Verification items for this drawing (mm, ordinates from the low corner). Give positions to 0.01 mm unless a question says otherwise; leave off trailing zeros. Loops run counter-clockwise (first coordinate to the right, second up) from the corner with the lowest first, then second, coordinate; pieces in that order, holes last. Notation, with made-up numbers: M 1,44 L 29,44 A15 ccw 29,68 Z; hole C 48.5,14.25 d7. An arc over 180 degrees is marked long. Use one line per item in the form item = value.
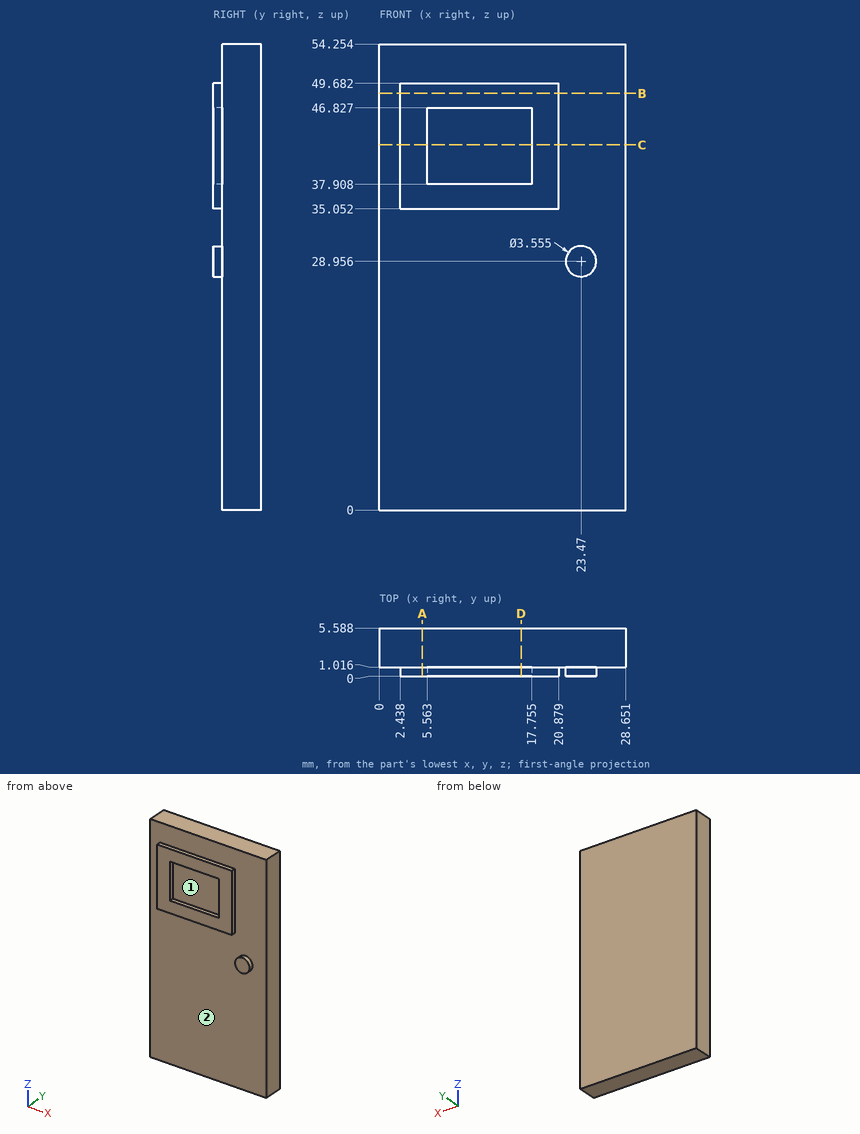
1) Section check C-C (z = 42.5). Record the cut outline in (x, y) (1 decimal), then the cut area to 3 significant figures.
Evaluation:
outline = M 0,1 L 2.4,1 L 2.4,0 L 5.6,0 L 5.6,1 L 17.8,1 L 17.8,0 L 20.9,0 L 20.9,1 L 28.7,1 L 28.7,5.6 L 0,5.6 Z
area = 137 mm^2
2) Scan lines: line 1 (Z direction, x = 9, y = 0.95); line 2 (Y direction, x = 8.25, z = 31); line 3 (X direction, y = 0.5, z = 40) (1 decimal). Record each from-to range of solid material in increasing order.
Evaluation:
line_1 = 35.05 to 37.91, 46.83 to 49.68
line_2 = 1.02 to 5.59
line_3 = 2.4 to 5.6, 17.8 to 20.9
3) Section check B-B (z = 48.5). Record the cut outline in (x, y), then the cut area to 3 significant figures.
Evaluation:
outline = M 0,1.02 L 2.44,1.02 L 2.44,0 L 20.88,0 L 20.88,1.02 L 28.65,1.02 L 28.65,5.59 L 0,5.59 Z
area = 150 mm^2
4) Depth check by flat-ended pin: pin 1 Ø0.5 at (y, z) = (0.5, 43.5) entering from -X; pin 2 Ø14.5 at (x, z) = (14.5, 27.5) entering from -Y; pin 3 Ø0.5 at (y, z) = (0.5, 41.5) entering from +X. Enter the tip coordinate at first touch or a pass-through.
Evaluation:
pin_1 = 2.44
pin_2 = 1.02
pin_3 = 20.88
5) Section check A-A (x = 5). Record the cut outline in (y, z) (1 decimal).
Evaluation:
outline = M 0,35.1 L 1,35.1 L 1,0 L 5.6,0 L 5.6,54.3 L 1,54.3 L 1,49.7 L 0,49.7 Z
6) Release check for a two-part mould opening along Z. For the marked faces 1 and 2 record: pulls with the +Z half, pulls with the -Z half, needs draft (parallel to the pull), parting line crosses it, or undercut.
Evaluation:
face_1 = undercut
face_2 = needs draft
7) Section check D-D (x = 16.5). Record the cut outline in (y, z) (1 decimal), then the cut area to 3 significant figures.
Evaluation:
outline = M 0,35.1 L 1,35.1 L 1,0 L 5.6,0 L 5.6,54.3 L 1,54.3 L 1,49.7 L 0,49.7 L 0,46.8 L 1,46.8 L 1,37.9 L 0,37.9 Z
area = 254 mm^2
